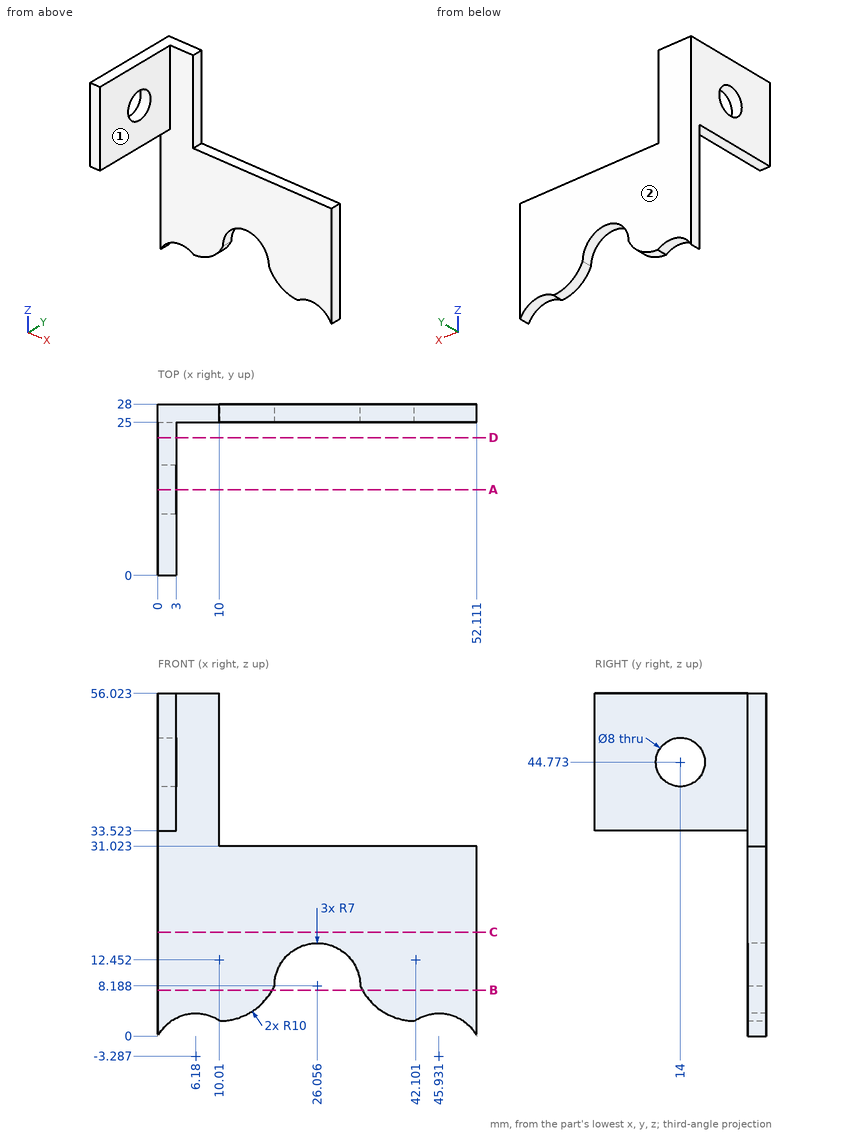
Drawing for the job (mm, zero at the part's lowest x, y, z). A direction names the side the tool comes from. Round coordinates to 2 decimals unless told otherwise and drop trailing zeros. Order: outer loops, then holes, each group sorted by start corner. A loop starts at its lowest first (then second) coordinate and runs counter-clockwise, first axis right, second up. Notation, with made-up numbers: (52.25, 9.5) -> (81.25, 9.5) arc R20 ccw to (81.25, 25.5) -> close; hole circle Ø4 at (-22, 35). An arc over 180 degrees is marked (long way). Put each result on its own line as item: value.
Q1. Tool access for the marked faces 1 and 2: list every direction of +Z, -Z, +X, -X, +Y, -Y with a clear straight run to the whole face (end or side of a thin tool).
From the geometry:
face 1: +Z, -Z, +X, -Y
face 2: +Z, -Z, +X, -X, +Y
Q2. Band-saw the part on C-C (z = 17). Give the cut face in (x, y), and give its area (3 significant figures).
From the geometry:
outline: (0, 25) -> (52.11, 25) -> (52.11, 28) -> (0, 28) -> close
area: 156 mm2
Q3. Wall check: line 1 (X direction, y = 14.5, z = 37.5); line 2 (Y direction, x = 44.5, z = 28); line 3 (Z direction, x = 41.5, y = 25.5). Give the ranges that are in metal, low to high. Write a range as [from, to].
From the geometry:
line 1: x = [0, 3]
line 2: y = [25, 28]
line 3: z = [2.47, 31.02]
Q4. Band-saw the part on A-A (y = 14). Give the cut face in (x, z), and give its area (3 significant figures).
From the geometry:
outline: (0, 33.52) -> (3, 33.52) -> (3, 40.77) -> (0, 40.77) -> close; (0, 48.77) -> (3, 48.77) -> (3, 56.02) -> (0, 56.02) -> close
area: 43.5 mm2
Q5. Band-saw the part on D-D (y = 22.5). Give the cut face in (x, z), and give its area (3 significant figures).
From the geometry:
outline: (0, 33.52) -> (3, 33.52) -> (3, 56.02) -> (0, 56.02) -> close
area: 67.5 mm2
Q6. Band-saw the part on B-B (z = 7.5). Give the cut face in (x, y), and give its area (3 significant figures).
From the geometry:
outline: (0, 25) -> (18.7, 25) -> (18.7, 28) -> (0, 28) -> close; (33.41, 25) -> (52.11, 25) -> (52.11, 28) -> (33.41, 28) -> close
area: 112 mm2
Q7. Pin check, flat tips, straight feed: pin 1 Ø2.5 at (y, z) = (26, 37.5) entering from +X; pin 2 Ø12 at (y, z) = (11.5, 31) entering from +X; pin 3 Ø2.5 at (x, y) = (23, 26) entering from +Z. Stop position of each tip, or through.
From the geometry:
pin 1: stops at x = 10
pin 2: stops at x = 3
pin 3: stops at z = 31.02
